Design review of the part shown in the three views and the two pictorial views. Dimensions are in mm from the part's minimum x, y and z. A direction names the side the tool comes from. Coordinates: 2 decimals unless noted, no trailing zeros. Order: outer loops, then holes, each group sorted by start corner. A loop starts at its lowest first (then second) coordinate and runs counter-clockwise, first axis right, second up. Notation, with made-up numbers: (63, 81) -> (88, 81) arc R18 cw to (88, 91) -> close; hole circle Ø6 at (-39, 67.5). An arc over 180 degrees is marked (long way). Write item = value, one per line. Start each with the question number.
1) Consider section B-B on z = 15. Give the boundary of the cut face in (x, y).
2) Wall thickness on probe 1 along Z at (x, y) = (18.5, 57.2); probe 2 along Z at (x, y) = (18, 57) (1 decimal); probe 3 along X at (y, z) = (57, 26) (1 decimal): over which ranges is each line inside the solid? List them lowest first. Write a range as [from, to].
3) Insertion check: pin 1 Ø3.5 at (x, y) = (18, 71) entering from -Z; pin 2 Ø4 at (x, z) = (5.08, 26.25) entering from -Y; pin 3 Ø0.9 at (x, z) = (5.5, 26.5) entering from +Y; pin 4 Ø3 at (y, z) = (31.5, 6.5) entering from +X. Each pin has a flat end and moves straight along its axis. Give the tip position at first contact, or say it passes through.
4) Consider section C-C on y = 53. Give the boundary of the cut face in (x, z), and give its area (3 significant figures).
5) Consider section D-D on x = 32.5. Give the boundary of the cut face in (y, z) (1 decimal).
6) Consider section A-A on x = 18.5. Give the boundary of the cut face in (y, z), and give its area (3 significant figures).
7) Machinability: for the marked faces 1 and 2, which of the approach directions +Z, -Z, +X, -X, +Y, -Y give a long, thin tool a straight path to every point of the face, cutting with its end or side? Answer none if there is none.
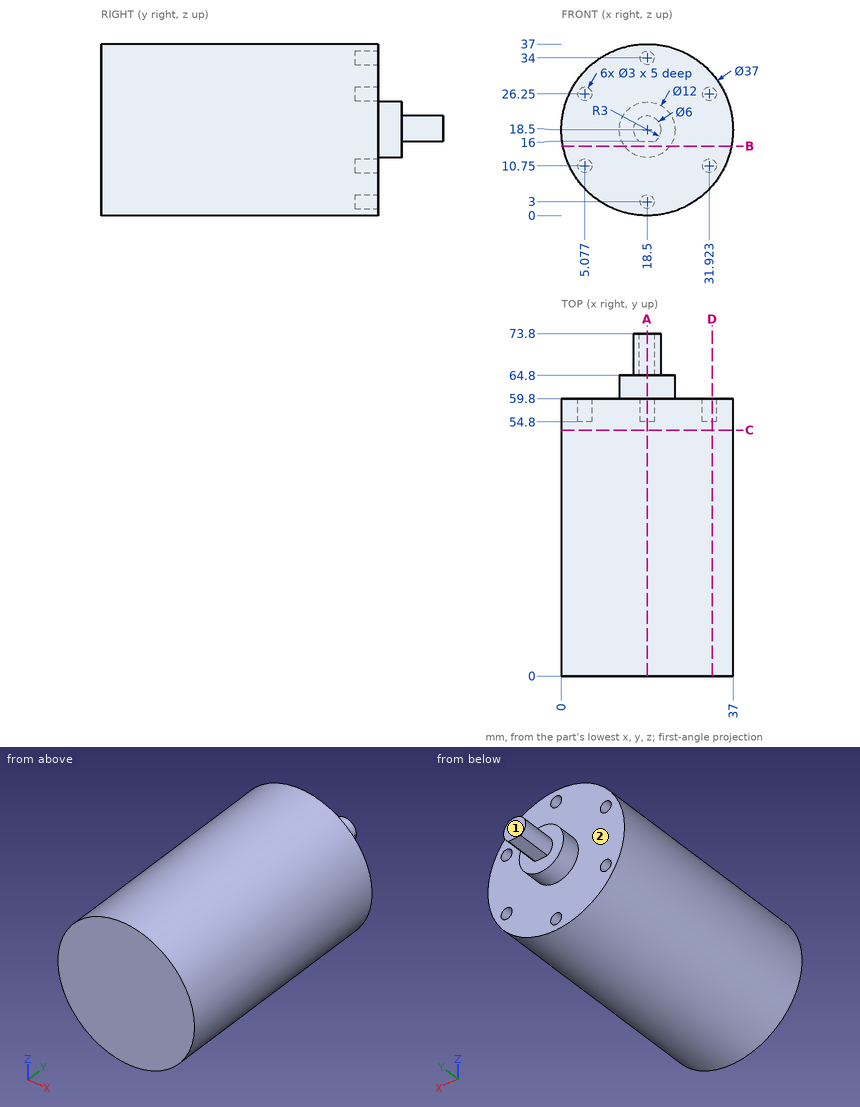
Answer sheet:
q1.outline = (0.33, 0) -> (36.67, 0) -> (36.67, 59.8) -> (23.37, 59.8) -> (23.37, 64.8) -> (13.63, 64.8) -> (13.63, 59.8) -> (0.33, 59.8) -> close
q2.probe_1 = [0, 1.5], [4.5, 32.5], [35.5, 37]
q2.probe_2 = [0, 1.6], [4.4, 32.6], [35.4, 37]
q2.probe_3 = [1.6, 3.6], [6.6, 30.4], [33.4, 35.4]
q3.pin_1 = 16
q3.pin_2 = 0
q3.pin_3 = 54.8
q3.pin_4 = 33.73
q4.outline = circle Ø37 at (18.5, 18.5)
q4.area = 1,080 mm2
q5.outline = (0, 6.4) -> (59.8, 6.4) -> (59.8, 9.4) -> (54.8, 9.4) -> (54.8, 12.1) -> (59.8, 12.1) -> (59.8, 24.9) -> (54.8, 24.9) -> (54.8, 27.6) -> (59.8, 27.6) -> (59.8, 30.6) -> (0, 30.6) -> close
q6.outline = (0, 0) -> (59.8, 0) -> (59.8, 1.5) -> (54.8, 1.5) -> (54.8, 4.5) -> (59.8, 4.5) -> (59.8, 12.5) -> (64.8, 12.5) -> (64.8, 16) -> (73.8, 16) -> (73.8, 21.5) -> (64.8, 21.5) -> (64.8, 24.5) -> (59.8, 24.5) -> (59.8, 32.5) -> (54.8, 32.5) -> (54.8, 35.5) -> (59.8, 35.5) -> (59.8, 37) -> (0, 37) -> close
q6.area = 2,290 mm2
q7.face_1 = +Z, -Z, +X, -X, +Y
q7.face_2 = +Y
